Design review of the part built by this model. Coordinates are the model's own, in mm. A direction names the side the tool comes from. Give positions to 0.01 mm unless a question says otherwise; leave off trailing zeros. Loops run counter-clockwise (first coordinate to the right, second up) from the corner with the lowest first, then second, coordinate; pieces in that order, holes last. Notation, with made-up numbers: (-24, 20.25) -> (-4, 20.25) arc R28 cw to (-4, 50.25) -> close; hole circle Ø10 at (-14.5, 11.25). An arc over 180 degrees is marked (long way). Answer as CSV lines item,"result".
Autodesk Inventor part; units mm, degrees
ref_plane "YZ Plane" through (0, 0, 0) normal (1, 0, 0) x (0, 1, 0)
ref_plane "XZ Plane" through (0, 0, 0) normal (0, 1, 0) x (-1, 0, 0)
ref_plane "XY Plane" through (0, 0, 0) normal (0, 0, 1) x (1, 0, 0)
sketch "Sketch1" plane through (0, 0, 0) normal (0, 1, 0) x (-1, 0, 0)
  circle A0 centre (0, 0) radius 14
  circle A1 centre (0, 0) radius 12
  dimension "d0" = 28
  dimension "d1" = 2
extrude "Extrusion1" add sketch "Sketch1" along normal blind 2
sketch "Sketch2" plane through (0, 0, 0) normal (0, -1, 0) x (1, 0, 0)
  line L0 (0, 0) -> (0, -37) construction
  arc A0 (9.1985, -10.5541) -> (-9.1985, -10.5541) centre (0, -37) ccw
  line L1 (0, 0) -> (0, 37) construction
  arc A1 (-9.1985, 10.5541) -> (9.1985, 10.5541) centre (0, 37) ccw
  line L2 (-13.0767, 5) -> (-9.0767, 5)
  line L3 (-9.0767, 5) -> (-9.0767, -5)
  line L4 (-9.0767, -5) -> (-13.0767, -5)
  line L5 (-7.8662, 0) -> (-7.8662, -5) construction
  arc A2 (9.1985, -10.5541) -> (9.1985, 10.5541) centre (0, 0) ccw
  arc A3 (-9.1985, 10.5541) -> (-13.0767, 5) centre (0, 0) ccw
  arc A4 (-13.0767, -5) -> (-9.1985, -10.5541) centre (0, 0) ccw
  line L6 (0, 0) -> (-9.0767, 0)
  dimension "d8" = 56
  dimension "d10" = 37
  dimension "d11" = 5
  dimension "d12" = 4
extrude "Extrusion2" add sketch "Sketch2" along normal blind 3
sketch "Sketch3" plane through (0, -3, 0) normal (0, -1, 0) x (1, 0, 0)
  circle A0 centre (0, 0) radius 1.5
  dimension "d15" = 3
extrude "Extrusion3" cut sketch "Sketch3" against normal through all
chamfer "Chamfer1" distance 2.8 angle 45 3 edges at (-11.4786, -3, -8.0151) (-11.4786, -3, 8.0151) (14, -3, 0)
sketch "Sketch4" plane through (0, 0, 0) normal (0, 1, 0) x (1, 0, 0)
  circle A0 centre (0, 0) radius 1.5
  circle A1 centre (0, 0) radius 11
  dimension "d21" = 22
  dimension "d22" = 3
extrude "Extrusion4" add sketch "Sketch4" along normal blind 18
sketch3d "Sketch6"
sketch " Sketch6" plane through (0, -3, 0) normal (0, -1, 0) x (1, 0, 0)
  line L0 (-6.7175, 6.7175) -> (6.7175, -6.7175) construction
  line L1 (5.6569, 5.6569) -> (-5.6569, -5.6569) construction
  circle A0 centre (-5.6569, -5.6569) radius 1.15
  circle A1 centre (6.7175, -6.7175) radius 1.15
  circle A2 centre (-6.7175, 6.7175) radius 1.15
  circle A3 centre (5.6569, 5.6569) radius 1.15
  circle A4 centre (0, 0) radius 1.5 construction
  line L2 (0, 0) -> (31.4092, 0) construction
extrude "Extrusion5" cut sketch " Sketch6" against normal up to surface (3 mm away)
properties part number "BrushlessInner"
Q1. We need section A-A, the plane x = 0. State the section outline as (y, z) points, and give its area (3 significant figures).
Filled sheet:
outline,"(-3, -9) -> (0, -9) -> (0, -11) -> (18, -11) -> (18, -1.5) -> (-3, -1.5) -> close; (-3, 1.5) -> (18, 1.5) -> (18, 11) -> (0, 11) -> (0, 9) -> (-3, 9) -> close; (0, -14) -> (2, -14) -> (2, -12) -> (0, -12) -> close; (0, 12) -> (2, 12) -> (2, 14) -> (0, 14) -> close"
area,"395 mm^2"
Q2. We need section B-B, the plane z = 0. State the section outline as (x, y) points.
Filled sheet:
outline,"(-14, 0) -> (-12, 0) -> (-12, 2) -> (-14, 2) -> close; (-11, 0) -> (-9.08, 0) -> (-9.08, -3) -> (-1.5, -3) -> (-1.5, 18) -> (-11, 18) -> close; (1.5, -3) -> (11.2, -3) -> (14, -0.2) -> (14, 2) -> (12, 2) -> (12, 0) -> (11, 0) -> (11, 18) -> (1.5, 18) -> close"
Q3. To check wall thickness, follow probe 1 along X at (y, z) = (1.65, 0); probe 2 along Z at (x, y) = (0, 13.75). State the ranges of each line that lie inside material, in increasing order. Write a range as from..to.
Filled sheet:
probe 1,"x = -14..-12, -11..-1.5, 1.5..11, 12..14"
probe 2,"z = -11..-1.5, 1.5..11"
Q4. We need section C-C, the plane x = -5. State the section outline as (y, z) points, and give its area (3 significant figures).
Filled sheet:
outline,"(-3, -9.45) -> (0, -9.45) -> (0, -9.8) -> (18, -9.8) -> (18, 9.8) -> (0, 9.8) -> (0, 9.45) -> (-3, 9.45) -> (-3, -4.71) -> (0, -4.71) -> (0, -6.6) -> (-3, -6.6) -> close; (0, -13.08) -> (2, -13.08) -> (2, -10.91) -> (0, -10.91) -> close; (0, 10.91) -> (2, 10.91) -> (2, 13.08) -> (0, 13.08) -> close"
area,"412 mm^2"
Q5. We need section D-D, the plane y = 9.5. State the section outline as (x, z) points, and give its area (3 significant figures).
Filled sheet:
outline,"circle Ø22 at (0, 0); hole circle Ø3 at (0, 0)"
area,"373 mm^2"
Q6. The part is to be moulded in two halves that separate along X. For faces 6 (the flat face through (0, 0, 10)), 7 (the flat face through (-13, 0, 0)), 8 (the conical face through (-9.635, -1.58, -8.15)), say which applies: pulls with the +X half, pulls with the -X half, needs draft (parallel to the pull), parting line crosses it, or undercut.
Filled sheet:
face 6,"undercut"
face 7,"needs draft"
face 8,"pulls with the -X half"
Q7. For faces 1 (the flat face through (-10, 0, 0)), 2 (the cylindrical face through (-12.932, 0.986, 5.362)), 3 (the flat face through (6.3, 2, 10.4)), 4 (the flat face through (0, 0, -10)), 5 (the cylindrical face through (-6.504, -1.521, -4.88)), list the 3-axis set-ups (+Z, -Z, +X, -X, +Y, -Y) from which the entire face can be reached by the end or side of a thin tool; tool diameter is ignored.
Filled sheet:
face 1,"-X, -Y"
face 2,"+Y, -Y"
face 3,"+Y"
face 4,"-Z, -Y"
face 5,"-Y"
Q8. Clearance check with flat-ended pins moving along their axes: pin 1 Ø4.5 at (x, z) = (-3.5, -12.5) entering from -Y; pin 2 Ø2 at (y, z) = (1, 10.5) entering from +X; pin 3 Ø4 at (x, y) = (6, 10.5) entering from +Z. State where each tip first meets the part, or that it passes through.
Filled sheet:
pin 1,"stops at y = 0"
pin 2,"stops at x = 10.28"
pin 3,"stops at z = 10.25"
